Verification items for the finished model (mm, model axes). Face numbers are marked on the shaded views. A direction names the side the tool comes from. Give positions to 0.01 mm unless a question says otherwise; leave off trailing zeros. Order: outer loops, then holes, each group sorted by start corner. A loop starts at its lowest first (then second) coordinate and runs counter-clockwise, first axis right, second up. Notation, with made-up numbers: M 60,11 L 65,11 A24 ccw 65,30 Z; hole C 86.25,12.5 d11. An arc over 180 degrees is marked long. Answer as a JSON object with one key per item and string values.
```python
from build123d import *

# Parameters (mm, degrees)
PRISM005_DEPTH           = 23
PRISM005_ROLL_ANGLE      = 153.435058
PRISM005_PITCH_ANGLE     = 37.760957
PRISM005_PLACEMENT_ANGLE = 140.768627
PRISM006_DEPTH           = 5
PRISM006_ROLL_ANGLE      = 153.435058
PRISM006_PITCH_ANGLE     = 37.760957
PRISM006_PLACEMENT_ANGLE = 140.768627
CHAMFER005_SIZE          = 4
BOX013_W                 = 6
BOX013_H                 = 42.4
BOX013_DEPTH             = 10.2
CYLINDER004_R            = 2
CYLINDER004_DEPTH        = 42
CYLINDER004_ROLL_ANGLE   = 90
PAD004_DEPTH             = 37
BODY004_PITCH_ANGLE      = -45
CYLINDER001_R            = 4
CYLINDER001_DEPTH        = 44
CYLINDER002_R            = 24
CYLINDER002_DEPTH        = 44
PAD003_DEPTH             = 5.62
PRISM_DEPTH              = 20
PRISM_PLACEMENT_ANGLE    = 30
CHAMFER001_SIZE          = 10
THICKNESS_T              = 3
CYLINDER047_R            = 1.5
CYLINDER047_DEPTH        = 15
BOX030_W                 = 4
BOX030_H                 = 7
BOX030_DEPTH             = 22
CHAMFER003_SIZE2         = 4
CHAMFER003_SIZE          = 15
BOX029_W                 = 12
BOX029_H                 = 10
BOX029_DEPTH             = 14
BOX029_ROLL_ANGLE        = -45
CYLINDER046_R            = 4
CYLINDER046_DEPTH        = 21
BOX031_W                 = 4
BOX031_H                 = 7
BOX031_DEPTH             = 10
CHAMFER004_SIZE          = 5
ARRAY001_COUNT           = 6


with BuildPart() as obj1:
    # Prism005 → Prism005 (new body)
    with BuildSketch(Plane.XY):
        Polygon((10, 0), (5, 8.660254), (-5, 8.660254), (-10, 0), (-5, -8.660254), (5, -8.660254), align=None)
    extrude(amount=PRISM005_DEPTH)


with BuildPart() as obj1_1:
    # Prism005 roll: moved
    add(obj1.part.rotate(Axis((0, 0, 0), (1, 0, 0)), PRISM005_ROLL_ANGLE))


with BuildPart() as obj1_2:
    # Prism005 pitch: moved
    add(obj1_1.part.rotate(Axis((0, 0, 0), (0, 1, 0)), PRISM005_PITCH_ANGLE))


with BuildPart() as obj1_3:
    # Prism005 placement: moved
    add(obj1_2.part.moved(Location((-45.8, 0, 18))).rotate(Axis((-45.8, 0, 18), (0, 0, 1)), PRISM005_PLACEMENT_ANGLE))


with BuildPart() as obj2:
    # Prism006 → Prism006 (new body)
    with BuildSketch(Plane.XY):
        Polygon((12, 0), (6, 10.392305), (-6, 10.392305), (-12, 0), (-6, -10.392305), (6, -10.392305), align=None)
    extrude(amount=PRISM006_DEPTH)


with BuildPart() as obj2_1:
    # Prism006 roll: moved
    add(obj2.part.rotate(Axis((0, 0, 0), (1, 0, 0)), PRISM006_ROLL_ANGLE))


with BuildPart() as obj2_2:
    # Prism006 pitch: moved
    add(obj2_1.part.rotate(Axis((0, 0, 0), (0, 1, 0)), PRISM006_PITCH_ANGLE))


with BuildPart() as obj2_3:
    # Prism006 placement: moved
    add(obj2_2.part.moved(Location((-44.8, 0, 17))).rotate(Axis((-44.8, 0, 17), (0, 0, 1)), PRISM006_PLACEMENT_ANGLE))

    # Chamfer005
    chamfer005_edges = [obj2_3.edges().sort_by_distance(p)[0] for p in [
        (-37.451495, -4e-06, 24.348434),
        (-52.148505, 4e-06, 9.651566),
    ]]
    chamfer(chamfer005_edges, length=CHAMFER005_SIZE)


with BuildPart() as cubo010:
    # Box013 → Box013 (new body)
    with BuildSketch(Plane(origin=(44.7, -21.2, 0), x_dir=(1, 0, 0), z_dir=(0, 0, 1))):
        with Locations((3, 21.2)):
            Rectangle(BOX013_W, BOX013_H)
    extrude(amount=BOX013_DEPTH)


with BuildPart() as obj3:
    # Cylinder004 → Cylinder004 (new body)
    with BuildSketch(Plane.XY):
        Circle(CYLINDER004_R)
    extrude(amount=CYLINDER004_DEPTH)


with BuildPart() as obj3_1:
    # Cylinder004 roll: moved
    add(obj3.part.rotate(Axis((0, 0, 0), (1, 0, 0)), CYLINDER004_ROLL_ANGLE))


with BuildPart() as obj3_2:
    # Cylinder004 placement: moved
    add(obj3_1.part.moved(Location((-39, 21, 33))))


with BuildPart() as obj4:
    # Sketch004 → Pad004 (new body)
    with BuildSketch(Plane.XY):
        Polygon((-40.876069, 10), (-49.536323, 5), (-49.536323, -5), (-40.876069, -10), (-32.215815, -5), (-32.215815, 5), align=None)
    extrude(amount=PAD004_DEPTH)


with BuildPart() as obj4_1:
    # Body004 pitch: moved
    add(obj4.part.rotate(Axis((0, 0, 0), (0, 1, 0)), BODY004_PITCH_ANGLE))


with BuildPart() as obj4_2:
    # Body004 placement: moved
    add(obj4_1.part.moved(Location((0, 0, 103))))


with BuildPart() as obj5:
    # Cylinder001 → Cylinder001 (new body)
    with BuildSketch(Plane(origin=(19, 7, 0), x_dir=(1, 0, 0), z_dir=(0, 0, 1))):
        Circle(CYLINDER001_R)
    extrude(amount=CYLINDER001_DEPTH)


with BuildPart() as fusion002:
    # Cylinder002 → Cylinder002 (new body)
    with BuildSketch(Plane.XY):
        Circle(CYLINDER002_R)
    extrude(amount=CYLINDER002_DEPTH)

    # Fusion002: union obj5
    add(obj5.part)


with BuildPart() as obj6:
    # Sketch003 → Pad003 (new body)
    with BuildSketch(Plane.YZ):
        Polygon((-3, 0.536587), (3, 0.536587), (4.5, -3.263413), (-4.5, -3.263413), align=None)
    extrude(amount=PAD003_DEPTH)


with BuildPart() as obj6_1:
    # Body003 placement: moved
    add(obj6.part.moved(Location((45.85, 0, 5))))


with BuildPart() as tapa_superior_con_agujero_hexagonal:
    # Prism → Prism (new body)
    with BuildSketch(Plane.XY):
        Polygon((55, 0), (27.5, 47.631397), (-27.5, 47.631397), (-55, 0), (-27.5, -47.631397), (27.5, -47.631397), align=None)
    extrude(amount=PRISM_DEPTH)


with BuildPart() as tapa_superior_con_agujero_hexagonal_1:
    # Prism placement: moved
    add(tapa_superior_con_agujero_hexagonal.part.rotate(Axis((0, 0, 0), (0, 0, 1)), PRISM_PLACEMENT_ANGLE))

    # Chamfer001
    chamfer001_edges = [tapa_superior_con_agujero_hexagonal_1.edges().sort_by_distance(p)[0] for p in [
        (23.815699, 41.25, 20),
        (-23.815699, 41.25, 20),
        (-47.631397, 0, 20),
        (-23.815699, -41.25, 20),
        (23.815699, -41.25, 20),
        (47.631397, 0, 20),
    ]]
    chamfer(chamfer001_edges, length=CHAMFER001_SIZE)

    # Thickness
    thickness_openings = [tapa_superior_con_agujero_hexagonal_1.faces().sort_by_distance(p)[0] for p in [
        (0, 0, 0),
    ]]
    offset(amount=THICKNESS_T, openings=thickness_openings, kind=Kind.INTERSECTION)

    # Cut001: cut obj6
    add(obj6_1.part, mode=Mode.SUBTRACT)

    # Cut002: cut Fusion002
    add(fusion002.part, mode=Mode.SUBTRACT)

    # Cut004: cut obj4)
    add(obj4_2.part, mode=Mode.SUBTRACT)

    # Cut005: cut obj3)
    add(obj3_2.part, mode=Mode.SUBTRACT)

    # Cut009: cut Cubo010
    add(cubo010.part, mode=Mode.SUBTRACT)

    # Fusion011: union obj2
    add(obj2_3.part)

    # Cut016: cut obj1
    add(obj1_3.part, mode=Mode.SUBTRACT)


with BuildPart() as cilindro023:
    # Cylinder047 → Cylinder047 (new body)
    with BuildSketch(Plane(origin=(0, -46, 0), x_dir=(1, 0, 0), z_dir=(0, 0, 1))):
        Circle(CYLINDER047_R)
    extrude(amount=CYLINDER047_DEPTH)


with BuildPart() as chamfer003:
    # Box030 → Box030 (new body)
    with BuildSketch(Plane(origin=(-2, -43, 0), x_dir=(1, 0, 0), z_dir=(0, 0, 1))):
        with Locations((2, 3.5)):
            Rectangle(BOX030_W, BOX030_H)
    extrude(amount=BOX030_DEPTH)

    # Chamfer003
    chamfer003_edges = [chamfer003.edges().sort_by_distance(p)[0] for p in [
        (0, -36, 0),
    ]]
    chamfer003_side = chamfer003.faces().sort_by_distance((0, -36, 11))[0]
    chamfer(chamfer003_edges, length=CHAMFER003_SIZE, length2=CHAMFER003_SIZE2, reference=chamfer003_side)


with BuildPart() as cubo025:
    # Box029 → Box029 (new body)
    with BuildSketch(Plane.XY):
        with Locations((6, 5)):
            Rectangle(BOX029_W, BOX029_H)
    extrude(amount=BOX029_DEPTH)


with BuildPart() as cubo025_1:
    # Box029 roll: moved
    add(cubo025.part.rotate(Axis((0, 0, 0), (1, 0, 0)), BOX029_ROLL_ANGLE))


with BuildPart() as cubo025_2:
    # Box029 placement: moved
    add(cubo025_1.part.moved(Location((-7, -59, 20))))


with BuildPart() as cut014:
    # Cylinder046 → Cylinder046 (new body)
    with BuildSketch(Plane(origin=(0, -46, 0), x_dir=(1, 0, 0), z_dir=(0, 0, 1))):
        Circle(CYLINDER046_R)
    extrude(amount=CYLINDER046_DEPTH)

    # Cut014: cut Cubo025
    add(cubo025_2.part, mode=Mode.SUBTRACT)


with BuildPart() as tapa_superior:
    # Box031 → Box031 (new body)
    with BuildSketch(Plane(origin=(-2, -56, 6), x_dir=(1, 0, 0), z_dir=(0, 0, 1))):
        with Locations((2, 3.5)):
            Rectangle(BOX031_W, BOX031_H)
    extrude(amount=BOX031_DEPTH)

    # Chamfer004
    chamfer004_edges = [tapa_superior.edges().sort_by_distance(p)[0] for p in [
        (0, -56, 16),
    ]]
    chamfer(chamfer004_edges, length=CHAMFER004_SIZE)

    # Fusion010: union Chamfer003, Cut014
    add(chamfer003.part)
    add(cut014.part)

    # Cut015: cut Cilindro023
    add(cilindro023.part, mode=Mode.SUBTRACT)

    # Array001: tapa superior ×6 about axis
    array001_axis = Axis((0, 0, 0), (0, 0, 1))


with BuildPart() as tapa_superior_1:
    add(tapa_superior.part)
    for i in range(1, ARRAY001_COUNT):
        add(tapa_superior.part.rotate(array001_axis, i * 360 / ARRAY001_COUNT))

    # Fusion012: union tapa superior con agujero hexagonal
    add(tapa_superior_con_agujero_hexagonal_1.part)


solid = tapa_superior_1.part
```
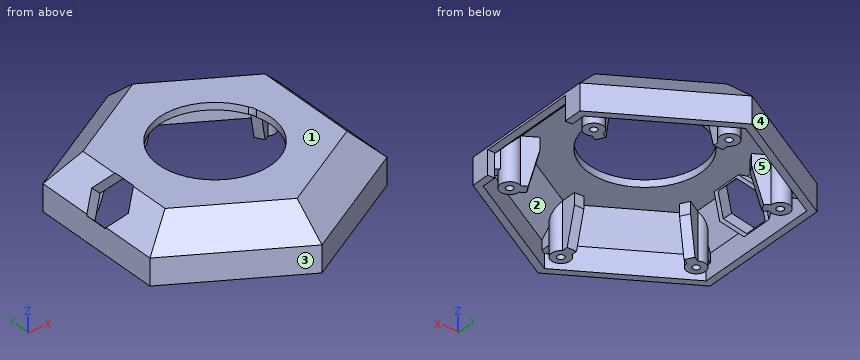
Q1. Tool access check on the marked faces 4 and 5. Record the directions out of +Z, -Z, +X, -X, +Y, -Y that give a thin tool (end or side, any length) a straight path to the whole face; none if there is none.
Resolved:
{"face 4": "+Z, -Z, -X, +Y", "face 5": "-Z"}
Q2. Section check A-A on x = 6. Record the cut outline in (y, z), then the cut area to 3 significant figures.
Resolved:
{"outline": "M -55,0 L -51.54,0 L -51.54,10 L -39.99,20 L -23.24,20 L -23.24,23 L -41.42,23 L -55,11.24 Z; M 23.24,20 L 39.99,20 L 51.54,10 L 51.54,0 L 55,0 L 55,11.24 L 41.42,23 L 23.24,23 Z", "area": "285 mm²"}
Q3. Material ranges on L1, parallel to X at y = 9.5, z = 15.25; L2, parallel to Y at x = -34, z = 9.5; L3, parallel to Y at x = 0.5, z = 4, recorded low to high.
Resolved:
{"L1": "x = -46.62 to -44.27, -41.83 to -39.48, 42.38 to 46.62", "L2": "y = -38.83 to -35.37, -21.94 to -17.32, 17.32 to 21.94, 35.37 to 38.83", "L3": "y = -58.18 to -54.71, -49.97 to -47.41, -44.59 to -38.93, 38.93 to 44.59, 47.41 to 49.97, 54.71 to 58.18"}
Q4. Gauge pin test, flat ends, axial feed: pin 1 Ø3.5 at (x, y) = (-39.5, -23) entering from -Z; pin 2 Ø2 at (y, z) = (-51.5, 11) entering from -X; pin 3 Ø1 at (x, z) = (11.5, 14) entering from +Y; pin 4 Ø3.5 at (y, z) = (-52.5, 8.5) entering from +X. Record the tip position at first contact, or that the pin passes through.
Resolved:
{"pin 1": "stops at z = 0", "pin 2": "stops at x = -13.79", "pin 3": "stops at y = 49.29", "pin 4": "stops at x = 13.36"}
Q5. Section check C-C on x = 27.5. Record the cut outline in (y, z).
Resolved:
{"outline": "M -42.59,0 L -39.12,0 L -39.12,10 L -27.58,20 L 27.58,20 L 39.12,10 L 39.12,0 L 42.59,0 L 42.59,11.24 L 29.01,23 L -29.01,23 L -42.59,11.24 Z"}
Q6. Section check B-B on z = 2. Count the separate pieces of the cut face and the enclosed holes in it, then the cut area to 3 significant figures.
Resolved:
{"separate pieces": "7", "enclosed holes": "6", "area": "1,220 mm²"}
Q7. Release check for a two-part mould opening along Y. For the marked faces 1, 2 and 3 record: +Y half, -Y half, draft (parallel to the pull), parting line (faces both ways), or undercut.
Resolved:
{"face 1": "draft", "face 2": "undercut", "face 3": "-Y half"}
